```python
from build123d import *

# Parameters (mm, degrees)
EXTRUDE_2_DEPTH     = 200
SKETCH_3_R          = 8
CUT_EXTRUDE_1_DEPTH = 175
SKETCH_4_W          = 30
SKETCH_4_H          = 15
CUT_EXTRUDE_2_DEPTH = 80
HOLE_WIZARD_M3_1_D  = 2.5


with BuildPart() as part:
    # 草图1 → 凸台-拉伸2 (new body)
    with BuildSketch(Plane(origin=(0, 0, 0), x_dir=(1, 0, 0), z_dir=(0, 1, 0))):
        Polygon((0, 0), (0, -25), (-10, -25), (-10, 15), (30, 15), (30, 0), align=None)
    extrude(amount=EXTRUDE_2_DEPTH)

    # 草图3 → 切除-拉伸1 (cut)
    with BuildSketch(Plane(origin=(0, 187.5, 0), x_dir=(1, 0, 0), z_dir=(0, 1, 0))):
        with Locations((15, 0)):
            Circle(SKETCH_3_R)
    extrude(amount=-CUT_EXTRUDE_1_DEPTH, mode=Mode.SUBTRACT)

    # 草图4 → 切除-拉伸2 (cut)
    with BuildSketch(Plane(origin=(0, 140, 0), x_dir=(1, 0, 0), z_dir=(0, 1, 0))):
        with Locations((15, 7.5)):
            Rectangle(SKETCH_4_W, SKETCH_4_H)
    extrude(amount=-CUT_EXTRUDE_2_DEPTH, mode=Mode.SUBTRACT)

    # M3 螺纹孔1 (through all)
    with Locations(Plane(origin=(0, 0, 0), x_dir=(0, 0, -1), z_dir=(1, 0, 0))):
        with Locations((-15, 140), (-15, 60)):
            Hole(HOLE_WIZARD_M3_1_D / 2)


solid = part.part
```
Input: part model. Units: mm. Frame: model coordinates. A direction names the side the tool comes from. Coordinates: 2 decimals unless noted, no trailing zeros. Write each loop counter-clockwise with the first axis right and the second up, starting at its lowest first coordinate (ties: lowest second). Pieces come first, ordered by that corner, then holes. Notation, with made-up numbers: (86, 55) -> (126, 55) arc R32 cw to (126, 83) -> close; hole circle Ø3 at (48.5, 56). An arc over 180 degrees is marked (long way). Write each question's results on one line, items separated by ' | '.
Item 1: Section query C-C on z = -6. Return loops of the section in (x, y), plus the area to 3 significant figures.
Conclusion:
outline: (-10, 0) -> (30, 0) -> (30, 60) -> (20.29, 60) -> (20.29, 12.5) -> (9.71, 12.5) -> (9.71, 60) -> (0, 60) -> (0, 140) -> (9.71, 140) -> (9.71, 187.5) -> (20.29, 187.5) -> (20.29, 140) -> (30, 140) -> (30, 200) -> (-10, 200) -> close | area: 4,590 mm^2
Item 2: Material intervals for probe 1 along Y at (x, z) = (-4.25, 15); probe 2 along Z at (x, y) = (-4.5, 140); probe 3 along Y at (x, z) = (10, -11), sorted ascending.
Conclusion:
probe 1: y = 0 to 58.75, 61.25 to 138.75, 141.25 to 200 | probe 2: z = -15 to 13.75, 16.25 to 25 | probe 3: y = 0 to 60, 140 to 200
Item 3: Pin query (flat end, axial travel): pin 1 Ø9 at (x, y) = (10, 19) entering from +Z; pin 2 Ø16.5 at (x, z) = (9, -7.5) entering from -Y; pin 3 Ø4 at (y, z) = (121.5, -0.5) entering from +X. Return the tip coordinate at first contact, or that it passes through.
Conclusion:
pin 1: stops at z = 0 | pin 2: stops at y = 0 | pin 3: stops at x = 0
Item 4: Section query B-B on y = 146.5. Return loops of the section in (x, z).
Conclusion:
outline: (-10, -15) -> (30, -15) -> (30, 0) -> (23, 0) arc R8 cw to (7, 0) -> (0, 0) -> (0, 25) -> (-10, 25) -> close
Item 5: Mould query, pull axis X, two halves, no side actions, for faces 1 (the flat face through (15, 140, -9)), 2 (the flat face through (15, 12.5, -3)), 3 (the flat face through (30, 170, -8)). Classes: +X half, -X half, draft (parallel to the pull), parting line (faces both ways), or undercut.
Conclusion:
face 1: draft | face 2: undercut | face 3: +X half
Item 6: Section query A-A on x = 15. Return loops of the section in (y, z).
Conclusion:
outline: (0, -15) -> (60, -15) -> (60, -8) -> (12.5, -8) -> (12.5, 0) -> (0, 0) -> close; (140, -15) -> (200, -15) -> (200, 0) -> (187.5, 0) -> (187.5, -8) -> (140, -8) -> close
Item 7: Set-up query: faces 4 (the flat face through (15, 60, -9)), 5 (the flat face through (6, 0, -4)), 6 (the flat face through (5, 23, 0)), 7 (the cylindrical face through (15, 37, -8)). Return all of +Z, -Z, +X, -X, +Y, -Y with unobstructed straight access to the full face (end or side cutting, diameter ignored); none if empty.
Conclusion:
face 4: +Z, -Z, +X | face 5: +Z, -Z, +X, -X, -Y | face 6: +Z, +X, +Y, -Y | face 7: +Z
Item 8: Section query D-D on x = 27. Return loops of the section in (y, z).
Conclusion:
outline: (0, -15) -> (60, -15) -> (60, 0) -> (0, 0) -> close; (140, -15) -> (200, -15) -> (200, 0) -> (140, 0) -> close
